```python
from build123d import *

# Parameters (mm, degrees)
FILLET1_R     = 0.5
CHAMFER1_SIZE = 0.5


with BuildPart() as part:
    # Sketch1 → Revolve1 (revolve)
    with BuildSketch(Plane.XY, mode=Mode.PRIVATE) as revolve1_sk:
        Polygon((0, 6), (0, 10), (4, 10), (4, 7.5), (31, 7.5), (31, 6), align=None)
    revolve(revolve1_sk.sketch.rotate(Axis((-6.114398422, 0, 0), (1, 0, 0)), 90), axis=Axis((-6.114398422, 0, 0), (1, 0, 0)))

    # Fillet1
    fillet1_edges = [part.edges().sort_by_distance(p)[0] for p in [
        (4, 0, -7.5),
    ]]
    fillet(fillet1_edges, radius=FILLET1_R)

    # Chamfer1
    chamfer1_edges = [part.edges().sort_by_distance(p)[0] for p in [
        (31, 0, -7.5),
        (0, 0, -10),
    ]]
    chamfer(chamfer1_edges, length=CHAMFER1_SIZE)


solid = part.part
```
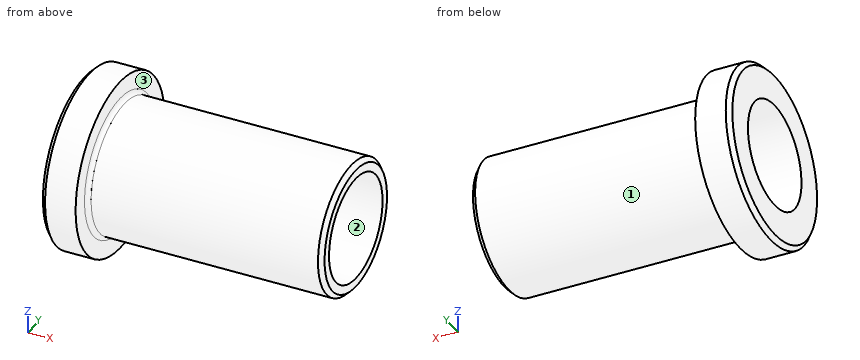
The model under review builds one solid part; all positions refer to its coordinate system, in mm. Face numbers are marked on the shaded views. Coordinates: 2 decimals unless noted, no trailing zeros. Write each loop counter-clockwise with the first axis right and the second up, starting at its lowest first coordinate (ties: lowest second). Pieces come first, ordered by that corner, then holes. Notation, with made-up numbers: (7, -29.5) -> (18, -29.5) arc R22 ccw to (18, -6.5) -> close; hole circle Ø11 at (-27, 55). An arc over 180 degrees is marked (long way). One line per item, written item: value. Start each with the question number.
Q1. Clearance check with flat-ended pins moving along their axes: P1, Ø6, axis at x = 14.5, z = 6, coming from the +Y side; P2, Ø5, axis at x = 16.5, z = 1, coming from the -Y side; P3, Ø5, axis at y = -7.5, z = 7.5, coming from the +X side. State where each tip first meets the part, or that it passes through.
Q2. To check wall thickness, follow probe 1 along Y at (x, z) = (19.5, 0); probe 2 along X at (y, z) = (-3.75, -8.25); probe 3 along Z at (x, y) = (9, -3). State the ranges of each line that lie inside material, in increasing order.
Q3. Add section C-C, the plane x = 25. Give the boundary of the cut face in (y, z), then the cut area to 3 significant figures.
Q4. The part is to be moulded in two halves that separate along Y. For the marked faces 1, 2 and 3, say which applies: +Y half, -Y half, draft (parallel to the pull), parting line (faces both ways), or undercut.
Q5. Add section A-A, the plane z = 0. Give the boundary of the cut face in (x, y), then the cut area to 3 significant figures.
Response:
1. P1: y = 6.87
1. P2: y = -7.5
1. P3: x = 4
2. probe 1: -7.5 to -6, 6 to 7.5
2. probe 2: 0 to 4
2. probe 3: -6.87 to -5.2, 5.2 to 6.87
3. outline: circle Ø15 at (0, 0); hole circle Ø12 at (0, 0)
3. area: 63.6 mm²
4. face 1: parting line
4. face 2: undercut
4. face 3: draft
5. outline: (0, -9.5) -> (0.5, -10) -> (4, -10) -> (4, -8) arc R0.5 cw to (4.5, -7.5) -> (30.5, -7.5) -> (31, -7) -> (31, -6) -> (0, -6) -> close; (0, 6) -> (31, 6) -> (31, 7) -> (30.5, 7.5) -> (4.5, 7.5) arc R0.5 cw to (4, 8) -> (4, 10) -> (0.5, 10) -> (0, 9.5) -> close
5. area: 113 mm²
